```python
from build123d import *

# Parameters (mm, degrees)
F0_W     = 7
F0_H     = 135
F1_DEPTH = 25
F3_DEPTH = 25
F4_W     = 25
F4_H     = 7.5
F5_DEPTH = 40
F7_R     = 5
F8_DEPTH = 7.501


with BuildPart() as f1:
    # F0 (on Front) → F1 (new body)
    with BuildSketch(Plane.XZ):
        with Locations((-31.12164, 8.253676)):
            Rectangle(F0_W, F0_H)
    extrude(amount=F1_DEPTH)

    # F2 (on face) → F3 (join)
    with BuildSketch(Plane.YZ.offset(-27.62164)):
        with BuildLine():
            ThreePointArc((-12.5, 75.753676), (-20.631728, 56.121948), (-1, 64.253676))
            ThreePointArc((-1, 64.253676), (-4.368272, 72.385404), (-12.5, 75.753676))
        make_face()
    extrude(amount=F3_DEPTH)

    # F4 (on face) → F5 (join)
    with BuildSketch(Plane.YZ.offset(-27.62164)):
        with Locations((-12.5, -55.496324)):
            Rectangle(F4_W, F4_H)
    extrude(amount=F5_DEPTH)

    # F7 (on face) → F8 (cut, through all)
    with BuildSketch(Plane.XY.offset(-51.746324)):
        with Locations((0, -12.5)):
            Circle(F7_R)
    extrude(amount=-F8_DEPTH, mode=Mode.SUBTRACT)


solid = f1.part
```
Could you check a few things on this model? Use its own coordinates, in mm. A direction names the side the tool comes from. Coordinates: 2 decimals unless noted, no trailing zeros. Write each loop counter-clockwise with the first axis right and the second up, starting at its lowest first coordinate (ties: lowest second). Pieces come first, ordered by that corner, then holes. Notation, with made-up numbers: M 77,-18.5 L 96,-18.5 A13 ccw 96,-11.5 Z; hole C -33,4 d1. An arc over 180 degrees is marked long. Answer as CSV lines item,"result". Start each with the question number.
1) For faces 1 (the flat face through (-8, -13, -51.746)), 2 (the flat face through (-2.622, -13, 64)), 3 (the flat face through (-11, -13, -59.246)), which set-ups out of +Z, -Z, +X, -X, +Y, -Y let a thin tool reach every point of the face, with its end or its side?
2) I want a section at A-A, the plane x = -26. Please give me the cut outline in (y, z), and give its area (3 significant figures).
3) I want a section at C-C, the plane y = -19.75. Please give me the cut outline in (x, z), and give its area (3 significant figures).
4) Please list where these lines run through material, in increasing order: line 1 (Y direction, x = 0, z = -54.75); line 2 (X direction, y = -8.25, z = 28.5); line 3 (Z direction, x = -17, y = -2). Write a range as from..to.
5) I want a section at B-B, the plane y = -10.5. Please give me the cut outline in (x, z), and give its area (3 significant figures).
6) For P1, Ø2, axis at x = -27.5, y = -13.5, coming from the +Z side; P2, Ø7, axis at y = -9.5, z = 62.5, coming from the +X side; P3, Ø7.5, axis at x = -12, y = -8, coming from the +Z side; P4, Ø7.5, axis at y = -11, z = 43.5, coming from the +X side, each with a flat end and sliding along its axis, tell me the tip position at first contact or that it passes through.
7) We'd pull the mould along X, two halves only. Please class faces 4 (the flat face through (-27.622, -12, -3)), 5 (the cylindrical face through (2.688, -8.284, -55.444)), 6 (the flat face through (-31, -12, 75.754)): +X half, -X half, draft (parallel to the pull), parting line (faces both ways), or undercut.
8) I want a section at D-D, the plane z = -9.5. Please give me the cut outline in (x, y), and give its area (3 significant figures).
Data:
1,face 1,"+X, +Y, -Y"
1,face 2,"+Z, +X, +Y, -Y"
1,face 3,"-Z, +X, -X, +Y, -Y"
2,outline,"M -25,-59.25 L 0,-59.25 L 0,-51.75 L -25,-51.75 Z; C -12.5,64.25 d23"
2,area,"603 mm^2"
3,outline,"M -34.62,-59.25 L 12.38,-59.25 L 12.38,-51.75 L -27.62,-51.75 L -27.62,55.33 L -2.62,55.33 L -2.62,73.18 L -27.62,73.18 L -27.62,75.75 L -34.62,75.75 Z"
3,area,"1,690 mm^2"
4,line 1,"y = -25..-17.5, -7.5..0"
4,line 2,"x = -34.62..-27.62"
4,line 3,"z = -59.25..-51.75, 59.56..68.94"
5,outline,"M -34.62,-59.25 L -4.58,-59.25 L -4.58,-51.75 L -27.62,-51.75 L -27.62,52.93 L -2.62,52.93 L -2.62,75.58 L -27.62,75.58 L -27.62,75.75 L -34.62,75.75 Z; M 4.58,-59.25 L 12.38,-59.25 L 12.38,-51.75 L 4.58,-51.75 Z"
5,area,"1,740 mm^2"
6,P1,"stops at z = 75.75"
6,P2,"stops at x = -2.62"
6,P3,"stops at z = 75.73"
6,P4,"stops at x = -27.62"
7,face 4,"+X half"
7,face 5,"undercut"
7,face 6,"draft"
8,outline,"M -34.62,-25 L -27.62,-25 L -27.62,0 L -34.62,0 Z"
8,area,"175 mm^2"
